Check sheet for the modelled part. Datum: model origin and axes. Units: mm. Round coordinates to 2 decimals unless told otherwise and drop trailing zeros. Loops run counter-clockwise (first coordinate to the right, second up) from the corner with the lowest first, then second, coordinate; pieces in that order, holes last. Notation, with made-up numbers: (-14.5, 18.5) -> (34.5, 18.5) arc R30 cw to (34.5, 44.5) -> close; hole circle Ø6 at (81, 83). An arc over 180 degrees is marked (long way). Use one line per item in the form item = value. Start each with the question number.
(1) Sectioned sample at B-B (x = 63.5). Record the cut outline in (y, z).
(2) Material ranges on probe 1 along Y at (x, z) = (12.7, 1.85); probe 2 along Y at (x, z) = (51, 3.4); probe 3 along Y at (x, z) = (88.9, 3.85), recorded low to high. Write a range as [from, to].
(3) Go/stop test with a flat-tipped pin: pin 1 (10 mm diameter, centred on x = 63.5, y = 39.55, fed in from +Z). Record where the tip stops, or that it passes through.
(4) Sectioned sample at D-D (x = 88.9). Record the cut outline in (y, z), and give its area (3 significant figures).
(5) Sectioned sample at C-C (z = 2.1). Record the cut outline in (x, y), and give its area (3 significant figures).
(6) Sectioned sample at A-A (x = 50.8). Record the cut outline in (y, z), and give its area (3 significant figures).
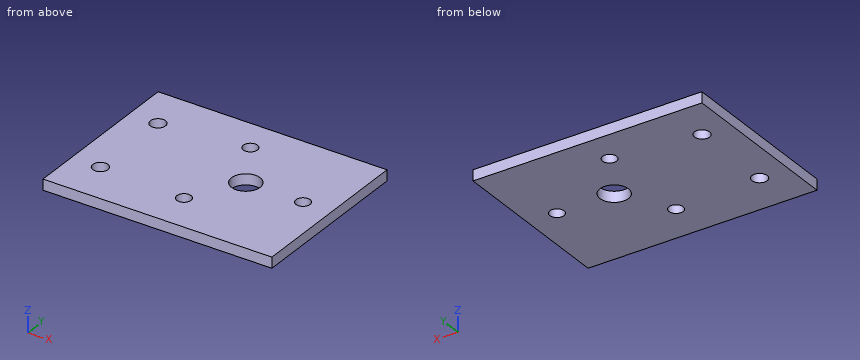
from build123d import *

# Parameters (mm, degrees)
SKETCH1_W           = 101.6
SKETCH1_H           = 76.2
BOSS_EXTRUDE1_DEPTH = 4.7625
SKETCH2_R           = 3.3782
CUT_EXTRUDE1_DEPTH  = 5.7625
SKETCH3_R           = 6.35
SKETCH3_R_2         = 3.1500064
CUT_EXTRUDE2_DEPTH  = 5.7625


with BuildPart() as part:
    # Sketch1 → Boss-Extrude1 (new body)
    with BuildSketch(Plane.XY):
        with Locations((50.8, 38.1)):
            Rectangle(SKETCH1_W, SKETCH1_H)
    extrude(amount=BOSS_EXTRUDE1_DEPTH)

    # Sketch2 → Cut-Extrude1 (cut, through all)
    with BuildSketch(Plane.XY.offset(4.7625)):
        with Locations((12.7, 57.15)):
            Circle(SKETCH2_R)
        with Locations((12.7, 19.05)):
            Circle(SKETCH2_R)
    extrude(amount=-CUT_EXTRUDE1_DEPTH, mode=Mode.SUBTRACT)

    # Sketch3 → Cut-Extrude2 (cut, through all)
    with BuildSketch(Plane.XY.offset(4.7625)):
        with Locations((63.5, 39.546877005)):
            Circle(SKETCH3_R)
        with Locations((50.8, 61.543922261)):
            Circle(SKETCH3_R_2)
        with Locations((88.9, 39.546877005)):
            Circle(SKETCH3_R_2)
        with Locations((50.8, 17.549831749)):
            Circle(SKETCH3_R_2)
    extrude(amount=-CUT_EXTRUDE2_DEPTH, mode=Mode.SUBTRACT)


solid = part.part
Checks:
q1.outline = (0, 0) -> (33.2, 0) -> (33.2, 4.76) -> (0, 4.76) -> close; (45.9, 0) -> (76.2, 0) -> (76.2, 4.76) -> (45.9, 4.76) -> close
q2.probe_1 = [0, 15.67], [22.43, 53.77], [60.53, 76.2]
q2.probe_2 = [0, 14.41], [20.69, 58.4], [64.69, 76.2]
q2.probe_3 = [0, 36.4], [42.7, 76.2]
q3.pin_1 = through
q4.outline = (0, 0) -> (36.4, 0) -> (36.4, 4.76) -> (0, 4.76) -> close; (42.7, 0) -> (76.2, 0) -> (76.2, 4.76) -> (42.7, 4.76) -> close
q4.area = 333 mm2
q5.outline = (0, 0) -> (101.6, 0) -> (101.6, 76.2) -> (0, 76.2) -> close; hole circle Ø6.76 at (12.7, 19.05); hole circle Ø6.76 at (12.7, 57.15); hole circle Ø6.3 at (50.8, 17.55); hole circle Ø6.3 at (50.8, 61.54); hole circle Ø12.7 at (63.5, 39.55); hole circle Ø6.3 at (88.9, 39.55)
q5.area = 7,450 mm2
q6.outline = (0, 0) -> (14.4, 0) -> (14.4, 4.76) -> (0, 4.76) -> close; (20.7, 0) -> (58.39, 0) -> (58.39, 4.76) -> (20.7, 4.76) -> close; (64.69, 0) -> (76.2, 0) -> (76.2, 4.76) -> (64.69, 4.76) -> close
q6.area = 303 mm2
